from build123d import *

# Parameters (mm, degrees)
SKETCH1_W           = 5
SKETCH1_H           = 1.5
BOSS_EXTRUDE1_DEPTH = 3
SKETCH2_W           = 10
SKETCH2_H           = 3
BOSS_EXTRUDE2_DEPTH = 34
SKETCH3_R           = 2.2
CUT_EXTRUDE1_DEPTH  = 38.871493237


with BuildPart() as part:
    # Sketch1 → Boss-Extrude1 (new body)
    with BuildSketch(Plane.XY):
        with Locations((2.5, 0.75)):
            Rectangle(SKETCH1_W, SKETCH1_H)
    extrude(amount=BOSS_EXTRUDE1_DEPTH)

    # Sketch2 → Boss-Extrude2 (add)
    with BuildSketch(Plane.XY.offset(3)):
        with Locations((2.5, 0.75)):
            Rectangle(SKETCH2_W, SKETCH2_H)
    extrude(amount=BOSS_EXTRUDE2_DEPTH)

    # Sketch3 → Cut-Extrude1 (cut, through all)
    with BuildSketch(Plane.XZ.offset(0.75)):
        with Locations(Location((2.5, 32.1, 0), (0, 0, 270))):
            Circle(SKETCH3_R)
    extrude(amount=-CUT_EXTRUDE1_DEPTH, mode=Mode.SUBTRACT)


solid = part.part
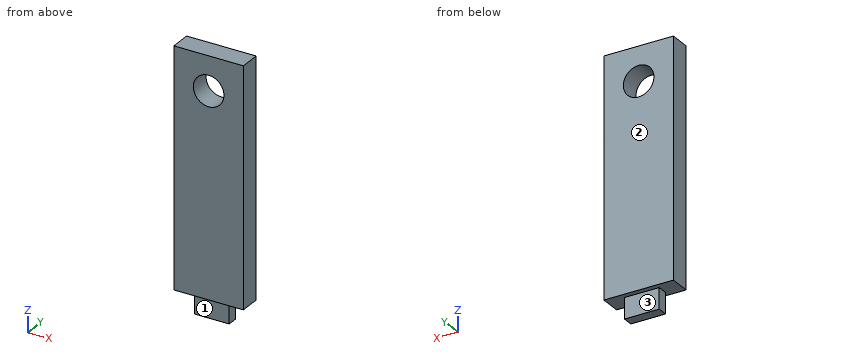
The listing builds one solid part. Answer for the finished solid, in the listing's coordinates (mm). Face numbers are marked on the shaded views. A direction names the side the tool comes from. Give positions to 0.01 mm unless a question says otherwise; leave off trailing zeros. Order: outer loops, then holes, each group sorted by start corner. A loop starts at its lowest first (then second) coordinate and runs counter-clockwise, first axis right, second up. Notation, with made-up numbers: (-2.75, 79.25) - (47.25, 79.25) arc R16 cw to (47.25, 99.25) - close; hole circle Ø8 at (-11, -7). An arc over 180 degrees is marked (long way). Use one line per item in the form item = value.
1) Each of these flat-tipped pins is pushed along its axis until it touches: pin 1 (1.2 mm diameter, centred on y = 0.5, z = 1, fed in from +X); pin 2 (0.8 mm diameter, centred on y = 1, z = 1, fed in from -X); pin 3 (0.9 mm diameter, centred on x = 1.5, z = 1.5, fed in from -Y). Where does it stop, or does it pass through?
Verdict:
pin_1 = 5
pin_2 = 0
pin_3 = 0
2) For the marked faces 1, 2 and 3, determine the directions among +Z, -Z, +X, -X, +Y, -Y from which every point of the face is accessible in a straight line to the end or side of a thin tool.
Verdict:
face_1 = -Z, +X, -X, -Y
face_2 = +Z, -Z, +X, -X, +Y
face_3 = -Z, +X, -X, +Y
3) Find section B-B on z = 32.1. Determine the outline of the cut face in (x, y).
Verdict:
outline = (-2.5, -0.75) - (0.3, -0.75) - (0.3, 2.25) - (-2.5, 2.25) - close; (4.7, -0.75) - (7.5, -0.75) - (7.5, 2.25) - (4.7, 2.25) - close
4) Find section C-C on y = 0.7. Determine the outline of the cut face in (x, z).
Verdict:
outline = (-2.5, 3) - (0, 3) - (0, 0) - (5, 0) - (5, 3) - (7.5, 3) - (7.5, 37) - (-2.5, 37) - close; hole circle Ø4.4 at (2.5, 32.1)
5) Consider probe 1 along X at (y, z) = (0.25, 32); probe 2 along Z at (x, y) = (4.25, 1.25); probe 3 along Z at (x, y) = (3, 1.1). Determine where each line is inside the solid, lowest interval first. Write a range as [from, to].
Verdict:
probe_1 = [-2.5, 0.3], [4.7, 7.5]
probe_2 = [0, 30.77], [33.43, 37]
probe_3 = [0, 29.96], [34.24, 37]
6) Find section D-D on x = 0.75. Determine the outline of the cut face in (y, z).
Verdict:
outline = (-0.75, 3) - (0, 3) - (0, 0) - (1.5, 0) - (1.5, 3) - (2.25, 3) - (2.25, 30.77) - (-0.75, 30.77) - close; (-0.75, 33.43) - (2.25, 33.43) - (2.25, 37) - (-0.75, 37) - close
7) Find section A-A on x = 2.5. Determine the outline of the cut face in (y, z).
Verdict:
outline = (-0.75, 3) - (0, 3) - (0, 0) - (1.5, 0) - (1.5, 3) - (2.25, 3) - (2.25, 29.9) - (-0.75, 29.9) - close; (-0.75, 34.3) - (2.25, 34.3) - (2.25, 37) - (-0.75, 37) - close
